The listing builds one solid part. Answer for the finished solid, in the listing's coordinates (mm). Face numbers are marked on the shaded views. A direction names the side the tool comes from. Round coordinates to 2 decimals unless told otherwise and drop trailing zeros. Loops run counter-clockwise (first coordinate to the right, second up) from the corner with the lowest first, then second, coordinate; pieces in that order, holes last. Notation, with made-up numbers: (32, 70) -> (75, 70) arc R15 ccw to (75, 75) -> close; hole circle Ø10 at (-13, 80). An arc over 180 degrees is marked (long way). Use a Markdown table: item, result. Add a question column.
Q1. Given pin 1 Ø3 at (x, z) = (-2.5, 4.5) entering from -Y; pin 2 Ø1 at (y, z) = (-82, 3) entering from -X; pin 3 Ø5 at (y, z) = (-210, 3.5) entering from +X; pin 4 Ø4 at (x, y) = (-18.5, -50) entering from +Z, each flat-ended and moving along its own axis, determine where each tip first touches the part or whether it passes through.
Q2. Section B-B on y = -183 is taken. Give the vertices of the cut face in (x, z).
Q3. Which of the six approach directions +Z, -Z, +X, -X, +Y, -Y give full straight-line access (tool end or side, diameter ignored) to the marked faces 1 and 2?
Q4. Section C-C on z = 1.75 is taken. Give the number of separate pieces and of enclosed holes in the cut face, then the cut area to 3 significant figures.
Q5. Section D-D on y = -146 is taken. Give the vertices of the cut face in (x, z).
Q6. Consider line 1 (X direction, y = -32, z = 1.75); line 2 (X direction, y = -74, z = 2); line 3 (X direction, y = -147.5, z = 6.25). Determine where each line is inside the solid, lowest interval first.
Q7. Section A-A on y = -111.5 is taken. Give the vertices of the cut face in (x, z), then the cut area to 3 significant figures.
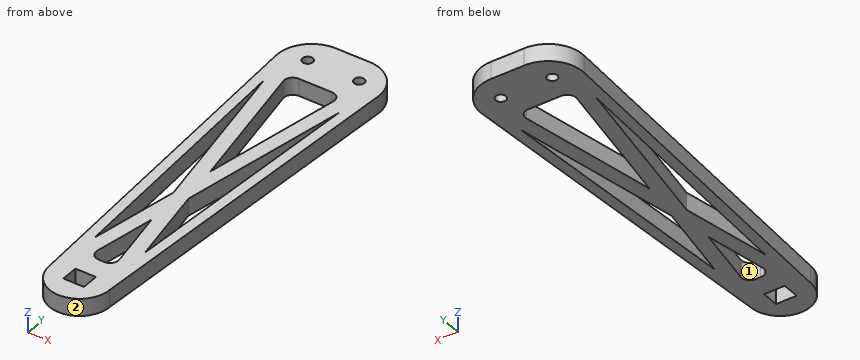
from build123d import *

# Parameters (mm, degrees)
SKETCH1_R           = 3
BOSS_EXTRUDE2_DEPTH = 10
FILLET1_R           = 20
FILLET2_R           = 20
CUT_EXTRUDE1_START  = -10
CUT_EXTRUDE1_DEPTH  = 10
FILLET3_R           = 5


with BuildPart() as part:
    # Sketch1 → Boss-Extrude2 (new body)
    with BuildSketch(Plane.XY):
        with BuildLine():
            Line((-30, 15.770412854), (-30, 0))
            Line((-30, 0), (-17.5, -210))
            ThreePointArc((-17.5, -210), (0, -227.5), (17.5, -210))
            Line((17.5, -210), (30, 0))
            Line((30, 0), (30, 15.770412854))
            Line((30, 15.770412854), (-30, 15.770412854))
        make_face()
        with Locations((-15, 0)):
            Circle(SKETCH1_R, mode=Mode.SUBTRACT)
        with Locations((15, 0)):
            Circle(SKETCH1_R, mode=Mode.SUBTRACT)
        Polygon((0, -205), (6, -205), (6, -215), (-6, -215), (-6, -205), align=None, mode=Mode.SUBTRACT)
    extrude(amount=BOSS_EXTRUDE2_DEPTH)

    # Fillet1
    fillet1_edges = [part.edges().sort_by_distance(p)[0] for p in [
        (-30, 15.770412854, 5),
    ]]
    fillet(fillet1_edges, radius=FILLET1_R)

    # Fillet2
    fillet2_edges = [part.edges().sort_by_distance(p)[0] for p in [
        (30, 15.770412854, 5),
    ]]
    fillet(fillet2_edges, radius=FILLET2_R)

    # Sketch4 → Cut-Extrude1 (cut)
    with BuildSketch(Plane.XY.offset(10).offset(CUT_EXTRUDE1_START)):
        Polygon((-15.651797422, -15), (0.190220551, -102.160979768), (15.643622882, -15), (15, -15), align=None)
        Polygon((-22.473027071, -25.6531452), (-13.367328465, -178.628881795), (-4.134156204, -126.551525408), align=None)
        Polygon((22.230419841, -27.161313899), (4.615986353, -126.511039477), (13.430162671, -175.005634359), align=None)
        with BuildLine():
            Line((0.291609598, -150.901585116), (-7.372445375, -194.128735111))
            ThreePointArc((-7.372445375, -194.128735111), (0.476576628, -192.506490497), (8.225632191, -194.553674383))
            Line((8.225632191, -194.553674383), (0.291609598, -150.901585116))
        make_face()
    extrude(amount=CUT_EXTRUDE1_DEPTH, mode=Mode.SUBTRACT)

    # Fillet3
    fillet3_edges = [part.edges().sort_by_distance(p)[0] for p in [
        (8.225632191, -194.553674383, 5),
        (-7.372445375, -194.128735111, 5),
        (-15.651797422, -15, 5),
        (15.643622882, -15, 5),
    ]]
    fillet(fillet3_edges, radius=FILLET3_R)


solid = part.part
Checked values:
| question | item | result |
|---|---|---|
| 1 | pin 1 | stops at y = -227.47 |
| 1 | pin 2 | stops at x = -25.15 |
| 1 | pin 3 | stops at x = 17.65 |
| 1 | pin 4 | stops at z = 10 |
| 2 | outline | (-19.11, 0) -> (-5.4, 0) -> (-5.4, 10) -> (-19.11, 10) -> close; (6.13, 0) -> (19.11, 0) -> (19.11, 10) -> (6.13, 10) -> close |
| 3 | face 1 | +Z, -Z |
| 3 | face 2 | +Z, -Z, -Y |
| 4 | separate pieces | 1 |
| 4 | enclosed holes | 7 |
| 4 | area | 7,590 mm2 |
| 5 | outline | (-21.31, 0) -> (-15.31, 0) -> (-15.31, 10) -> (-21.31, 10) -> close; (-7.58, 0) -> (8.16, 0) -> (8.16, 10) -> (-7.58, 10) -> close; (15.16, 0) -> (21.31, 0) -> (21.31, 10) -> (15.16, 10) -> close |
| 6 | line 1 | x = -28.1 to -22.1, -21.32 to -12.56, 12.63 to 21.37, 21.94 to 28.1 |
| 6 | line 2 | x = -25.6 to -19.6, -13.69 to -4.93, 5.18 to 13.93, 19.44 to 25.6 |
| 6 | line 3 | x = -21.22 to -15.22, -7.85 to 8.43, 15.07 to 21.22 |
| 7 | outline | (-23.36, 0) -> (-17.36, 0) -> (-17.36, 10) -> (-23.36, 10) -> close; (-6.87, 0) -> (7.28, 0) -> (7.28, 10) -> (-6.87, 10) -> close; (17.21, 0) -> (23.36, 0) -> (23.36, 10) -> (17.21, 10) -> close |
| 7 | area | 263 mm2 |
